Autodesk Inventor part; units mm, degrees
ref_plane "YZ Plane" through (0, 0, 0) normal (1, 0, 0) x (0, 1, 0)
ref_plane "XZ Plane" through (0, 0, 0) normal (0, 1, 0) x (-1, 0, 0)
ref_plane "XY Plane" through (0, 0, 0) normal (0, 0, 1) x (1, 0, 0)
sketch "Esquisse1" plane through (0, 0, 0) normal (1, 0, 0) x (0, 1, 0)
  line L0 (-15.5, -35.5) -> (15.5, -35.5)
  line L1 (15.5, -35.5) -> (15.5, 35.5)
  line L2 (15.5, 35.5) -> (-15.5, 35.5)
  line L3 (-15.5, 35.5) -> (-15.5, -35.5)
  line L4 (-15.5, -35.5) -> (15.5, 35.5) construction
  line L5 (15.5, -35.5) -> (-15.5, 35.5) construction
  point P0 (0, 0)
  dimension "d0" = 31
  dimension "d1" = 71
extrude "Extrusion1" add sketch "Esquisse1" against normal blind 6
sketch "Esquisse2" plane through (0, 0, 0) normal (1, 0, 0) x (0, 0, -1)
  line L0 (33.6, -13.6) -> (-33.6, -13.6)
  line L1 (-33.6, -13.6) -> (-33.6, 13.6)
  line L2 (-33.6, 13.6) -> (33.6, 13.6)
  line L3 (33.6, 13.6) -> (33.6, -13.6)
  line L4 (33.6, -13.6) -> (-33.6, 13.6) construction
  line L5 (-33.6, -13.6) -> (33.6, 13.6) construction
  point P0 (0, 0)
  dimension "d4" = 67.2
  dimension "d5" = 27.2
extrude "Extrusion2" cut sketch "Esquisse2" against normal blind 3
sketch "Esquisse3" plane through (0, 0, 0) normal (1, 0, 0) x (0, 0, -1)
  line L0 (32, -12) -> (-32, 12) construction
  line L1 (-32, -12) -> (32, 12) construction
  arc A0 (-30.0791, 13.6) -> (-33.6, 10.0791) centre (-32, 12) ccw
  arc A1 (33.5, 10) -> (30, 13.5) centre (32, 12) ccw
  arc A2 (30.0791, -13.6) -> (33.6, -10.0791) centre (32, -12) ccw
  line L2 (-33.6, 13.6) -> (33.6, 13.6)
  line L3 (33.6, -13.6) -> (-33.6, 13.6) construction
  line L4 (-33.5, -13.5) -> (33.5, 13.5) construction
  arc A3 (-33.5, -10) -> (-30, -13.5) centre (-32, -12) ccw
  line L5 (-33.6, 13.6) -> (-30.0791, 13.6)
  line L6 (30, 13.5) -> (33.5, 13.5)
  line L7 (-33.5, -13.5) -> (-33.5, -10)
  line L8 (-33.6, 10.0791) -> (-33.6, 13.6)
  line L9 (33.6, -13.6) -> (30.0791, -13.6)
  line L10 (-30, -13.5) -> (-33.5, -13.5)
  line L11 (33.5, 13.5) -> (33.5, 10)
  line L12 (33.6, -10.0791) -> (33.6, -13.6)
  point P0 (0, 0)
  point P1 (33.5, 13.5)
  point P2 (30.0791, 13.6)
  point P3 (-30.0791, 13.6)
  dimension "d8" = 64
  dimension "d9" = 24
  dimension "d10" = 5
  dimension "d12" = 5
  dimension "d13" = 5
extrude "Extrusion3" cut sketch "Esquisse3" against normal blind 3
sketch "Esquisse4" plane through (-6, 0, 0) normal (-1, 0, 0) x (0, 0, 1)
  line L0 (-28.9525, 9.2685) -> (3.8656, 9.2685) construction
  line L1 (3.8656, 9.2685) -> (3.8656, -1.9036) construction
  line L2 (3.8656, -1.9036) -> (-28.9525, -1.9036) construction
  line L3 (-28.9525, -1.9036) -> (-28.9525, 9.2685) construction
  line L4 (8.1238, -3.2547) -> (23.4156, -3.2547) construction
  line L5 (23.4156, -3.2547) -> (23.4156, -10.1675) construction
  line L6 (23.4156, -10.1675) -> (8.1238, -10.1675) construction
  line L7 (8.1238, -10.1675) -> (8.1238, -3.2547) construction
  line L8 (-28.297, 3.0616) -> (-28.297, 9.1616)
  line L9 (-28.297, 9.1616) -> (-25.9955, 9.1616)
  spline S0 degree 2 poles (-25.9955, 9.1616) (-25.3865, 9.1616) (-25.0657, 9.1012) knots 0 0 0 1 1 1
  spline S1 degree 2 poles (-25.0657, 9.1012) (-24.6147, 9.0268) (-24.0102, 8.6083) (-23.6383, 7.8505) (-23.6383, 7.3948) knots 0 0 0 1 2 3 3 3
  spline S2 degree 2 poles (-23.6383, 7.3948) (-23.6383, 6.6184) (-24.6286, 5.5397) (-25.9211, 5.5397) knots 0 0 0 1 2 2 2
  line L10 (-25.9211, 5.5397) -> (-27.488, 5.5397)
  line L11 (-27.488, 5.5397) -> (-27.488, 3.0616)
  line L12 (-27.488, 3.0616) -> (-28.297, 3.0616)
  line L13 (-27.488, 6.2604) -> (-25.9118, 6.2604)
  spline S3 degree 2 poles (-25.9118, 6.2604) (-25.1261, 6.2604) (-24.4705, 6.8416) (-24.4705, 7.3716) knots 0 0 0 1 2 2 2
  spline S4 degree 2 poles (-24.4705, 7.3716) (-24.4705, 7.7528) (-24.8564, 8.3015) (-25.1726, 8.3852) knots 0 0 0 1 2 2 2
  spline S5 degree 2 poles (-25.1726, 8.3852) (-25.3772, 8.441) (-25.9258, 8.441) knots 0 0 0 1 1 1
  line L14 (-25.9258, 8.441) -> (-27.488, 8.441)
  line L15 (-27.488, 8.441) -> (-27.488, 6.2604)
  line L16 (-18.2589, 5.205) -> (-17.45, 5.0004)
  spline S6 degree 2 poles (-17.45, 5.0004) (-17.7057, 4.0054) (-19.0214, 2.9593) (-19.9746, 2.9593) knots 0 0 0 1 2 2 2
  spline S7 degree 2 poles (-19.9746, 2.9593) (-20.9602, 2.9593) (-22.197, 3.7637) (-22.8432, 5.284) (-22.8432, 6.1581) knots 0 0 0 1 2 3 3 3
  spline S8 degree 2 poles (-22.8432, 6.1581) (-22.8432, 7.1112) (-22.1133, 8.5339) (-20.7696, 9.2685) (-19.9606, 9.2685) knots 0 0 0 1 2 3 3 3
  spline S9 degree 2 poles (-19.9606, 9.2685) (-19.0447, 9.2685) (-17.7987, 8.334) (-17.5522, 7.4925) knots 0 0 0 1 2 2 2
  line L17 (-17.5522, 7.4925) -> (-18.3473, 7.3019)
  spline S10 degree 2 poles (-18.3473, 7.3019) (-18.5612, 7.9667) (-19.3655, 8.5758) (-19.9792, 8.5758) knots 0 0 0 1 2 2 2
  spline S11 degree 2 poles (-19.9792, 8.5758) (-20.6813, 8.5758) (-21.6298, 7.9016) (-22.011, 6.7672) (-22.011, 6.1628) knots 0 0 0 1 2 3 3 3
  spline S12 degree 2 poles (-22.011, 6.1628) (-22.011, 5.3863) (-21.5554, 4.224) (-20.6022, 3.6521) (-20.0443, 3.6521) knots 0 0 0 1 2 3 3 3
  spline S13 degree 2 poles (-20.0443, 3.6521) (-19.3655, 3.6521) (-18.4263, 4.4332) (-18.2589, 5.205) knots 0 0 0 1 2 2 2
  line L18 (-17.1198, 3.0616) -> (-14.7766, 9.1616)
  line L19 (-14.7766, 9.1616) -> (-13.9025, 9.1616)
  line L20 (-13.9025, 9.1616) -> (-11.4104, 3.0616)
  line L21 (-11.4104, 3.0616) -> (-12.331, 3.0616)
  line L22 (-12.331, 3.0616) -> (-13.0377, 4.9074)
  line L23 (-13.0377, 4.9074) -> (-15.5948, 4.9074)
  line L24 (-15.5948, 4.9074) -> (-16.2644, 3.0616)
  line L25 (-16.2644, 3.0616) -> (-17.1198, 3.0616)
  line L26 (-15.3624, 5.563) -> (-13.2888, 5.563)
  line L27 (-13.2888, 5.563) -> (-13.9304, 7.2554)
  spline S14 degree 2 poles (-13.9304, 7.2554) (-14.2186, 8.0272) (-14.3581, 8.52) knots 0 0 0 1 1 1
  spline S15 degree 2 poles (-14.3581, 8.52) (-14.479, 7.9342) (-14.6882, 7.353) knots 0 0 0 1 1 1
  line L28 (-14.6882, 7.353) -> (-15.3624, 5.563)
  line L29 (8.0842, -9.3547) -> (10.1406, -3.2547)
  line L30 (10.1406, -3.2547) -> (11.1392, -3.2547)
  line L31 (11.1392, -3.2547) -> (13.1956, -9.3547)
  line L32 (13.1956, -9.3547) -> (12.3404, -9.3547)
  line L33 (12.3404, -9.3547) -> (11.7867, -7.6493)
  line L34 (11.7867, -7.6493) -> (9.4585, -7.6493)
  line L35 (9.4585, -7.6493) -> (8.9048, -9.3547)
  line L36 (8.9048, -9.3547) -> (8.0842, -9.3547)
  line L37 (11.5643, -6.9573) -> (10.6201, -4.0852)
  line L38 (10.6201, -4.0852) -> (9.6809, -6.9573)
  line L39 (9.6809, -6.9573) -> (11.5643, -6.9573)
  line L40 (18.2229, -9.3547) -> (17.17, -9.3547)
  line L41 (17.17, -9.3547) -> (14.9406, -6.5173)
  line L42 (14.9406, -6.5173) -> (14.5846, -6.9177)
  line L43 (14.5846, -6.9177) -> (14.5846, -9.3547)
  line L44 (14.5846, -9.3547) -> (13.7739, -9.3547)
  line L45 (13.7739, -9.3547) -> (13.7739, -3.2547)
  line L46 (13.7739, -3.2547) -> (14.5846, -3.2547)
  line L47 (14.5846, -3.2547) -> (14.5846, -6.0576)
  line L48 (14.5846, -6.0576) -> (17.0859, -3.2547)
  line L49 (17.0859, -3.2547) -> (18.0746, -3.2547)
  line L50 (18.0746, -3.2547) -> (15.5486, -5.9785)
  line L51 (15.5486, -5.9785) -> (18.2229, -9.3547)
  line L52 (18.0499, -9.3547) -> (20.1063, -3.2547)
  line L53 (20.1063, -3.2547) -> (21.1048, -3.2547)
  line L54 (21.1048, -3.2547) -> (23.1612, -9.3547)
  line L55 (23.1612, -9.3547) -> (22.306, -9.3547)
  line L56 (22.306, -9.3547) -> (21.7524, -7.6493)
  line L57 (21.7524, -7.6493) -> (19.4241, -7.6493)
  line L58 (19.4241, -7.6493) -> (18.8705, -9.3547)
  line L59 (18.8705, -9.3547) -> (18.0499, -9.3547)
  line L60 (21.5299, -6.9573) -> (20.5858, -4.0852)
  line L61 (20.5858, -4.0852) -> (19.6466, -6.9573)
  line L62 (19.6466, -6.9573) -> (21.5299, -6.9573)
  point P0 (0, 0)
extrude "Extrusion4" add sketch "Esquisse4" along normal blind 1
sketch "Esquisse5" plane through (-6, 0, 0) normal (-1, 0, 0) x (0, 0, 1)
  arc A0 (-30.0791, 13.6) -> (-33.6, 10.0791) centre (-32, 12) ccw
  line L0 (32, -12) -> (-32, -12)
  line L1 (-32, -12) -> (-32, 12)
  line L2 (-32, 12) -> (32, 12)
  line L3 (32, 12) -> (32, -12)
  line L4 (32, -12) -> (-32, 12) construction
  line L5 (-32, -12) -> (32, 12) construction
  circle A1 centre (-32, 12) radius 1.25
  circle A2 centre (-32, -12) radius 1.25
  circle A3 centre (32, 12) radius 1.25
  circle A4 centre (32, -12) radius 1.25
  line L6 (35.5, 15.5) -> (-35.5, 15.5)
  line L7 (35.5, -15.5) -> (35.5, 15.5)
  point P0 (0, 0)
  dimension "d18" = 64
  dimension "d19" = 24
  dimension "d20" = 2.5
  dimension "d21" = 2.5
  dimension "d22" = 2.5
  dimension "d24" = 2.5
hole "Perçage1" at (-6, 12, 32) at (-6, -12, -32) at (-6, -12, 32) at (-6, 12, -32) direction (1, 0, 0) diameter 2.5 end through all
sketch "Esquisse6" plane through (-6, 0, 0) normal (-1, 0, 0) x (0, 0, 1)
  circle A0 centre (21, 6) radius 1.8
  line L0 (35.5, 15.5) -> (-35.5, 15.5)
  line L1 (35.5, -15.5) -> (35.5, 15.5)
  point P0 (0, 0)
  dimension "d37" = 3.6
  dimension "d38" = 9.5
  dimension "d39" = 14.5
extrude "Extrusion5" cut sketch "Esquisse6" against normal blind 10
properties part number "wb_box2026_lid1"
The model under review builds one solid part; all positions refer to its coordinate system, in mm. A direction names the side the tool comes from. Give positions to 0.01 mm unless a question says otherwise; leave off trailing zeros. Loops run counter-clockwise (first coordinate to the right, second up) from the corner with the lowest first, then second, coordinate; pieces in that order, holes last. Notation, with made-up numbers: (65, 15) -> (99, 15) arc R29 ccw to (99, 44) -> close; hole circle Ø2 at (-27, 22). An arc over 180 degrees is marked (long way). Put each result on its own line as item: value. Start each with the question number.
1. We need section D-D on y = 0. State the section outline as (x, z) points.
2. We need section B-B on z = 32. State the section outline as (x, y) points, then the cut area to 3 significant figures.
3. We need section C-C on x = -2. State the section outline as (y, z) points, then the cut area to 3 significant figures.
4. Mouldability with a two-part tool opening along Y and no side actions: class faces 6 (the face through (-7, 6, -27)), 7 (the face through (-6.493, -6.347, 9.098)), 8 (the face through (-6.493, -4.598, 16.829)) as released by +Y, released by -Y, zero draft, split by the parting line, or undercut.
5. We need section A-A on y = -12. State the section outline as (x, z) points, then the cut area to 3 significant figures.
6. Wall thickness on probe 1 along Y at (x, z) = (-4.4, -32); probe 2 along Z at (x, y) = (-5.2, 12); probe 3 along Y at (x, z) = (-0.85, -32): over which ranges is each line inside the solid? List them lowest first.
7. For faces 1 (the face through (-1, 0, 33.6)), 2 (the face through (-6.493, -6.262, 12.153)), 3 (the face through (-4.479, -13.054, 32.672)), 4 (the face through (-6, 6, -14)), 5 (the face through (-6.493, -7.956, 16.071)), list the 3-axis set-ups (+Z, -Z, +X, -X, +Y, -Y) from which the entire face can be reached by the end or side of a thin tool; tool diameter is ignored.
8. Clearance check with flat-ended pins moving along their axes: P1, Ø0.8, axis at x = -6.5, z = 17.5, coming from the +Y side; P2, Ø3, axis at y = 12, z = -32, coming from the +X side; P3, Ø2, axis at y = -12, z = -32, coming from the +X side; P4, Ø5.5, axis at y = -12, z = -32, coming from the -X side. State where each tip first meets the part, or that it passes through.
Determined:
1. outline: (-6, -35.5) -> (0, -35.5) -> (0, -33.6) -> (-3, -33.6) -> (-3, 33.6) -> (0, 33.6) -> (0, 35.5) -> (-6, 35.5) -> close
2. outline: (-6, -15.5) -> (0, -15.5) -> (0, -14.5) -> (-3, -14.5) -> (-3, -13.25) -> (-6, -13.25) -> close; (-6, -10.75) -> (-3, -10.75) -> (-3, 10.75) -> (-6, 10.75) -> close; (-6, 13.25) -> (-3, 13.25) -> (-3, 14.5) -> (0, 14.5) -> (0, 15.5) -> (-6, 15.5) -> close
2. area: 84.0 mm^2
3. outline: (-15.5, -35.5) -> (15.5, -35.5) -> (15.5, 35.5) -> (-15.5, 35.5) -> close; hole (-13.6, -30.08) arc R2.5 ccw (long way) to (-10.08, -33.6) -> (10.08, -33.6) arc R2.5 ccw (long way) to (13.6, -30.08) -> (13.6, 30.08) arc R2.5 ccw (long way) to (10.08, 33.6) -> (-10.08, 33.6) arc R2.5 ccw (long way) to (-13.6, 30.08) -> close
3. area: 354 mm^2
4. face 6: zero draft
4. face 7: released by +Y
4. face 8: undercut
5. outline: (-6, -35.5) -> (0, -35.5) -> (0, -34.5) -> (-3, -34.5) -> (-3, -33.25) -> (-6, -33.25) -> close; (-6, -30.75) -> (-3, -30.75) -> (-3, 30.75) -> (-6, 30.75) -> close; (-6, 33.25) -> (-3, 33.25) -> (-3, 34.5) -> (0, 34.5) -> (0, 35.5) -> (-6, 35.5) -> close
5. area: 204 mm^2
6. probe 1: -15.5 to -13.25, -10.75 to 10.75, 13.25 to 15.5
6. probe 2: -35.5 to -33.25, -30.75 to 30.75, 33.25 to 35.5
6. probe 3: -15.5 to -14.5, 14.5 to 15.5
7. face 1: +X
7. face 2: -X, +Y
7. face 3: +X, -X
7. face 4: -X
7. face 5: -X, -Y
8. P1: y = -3.25
8. P2: x = -3
8. P3: through
8. P4: x = -6
